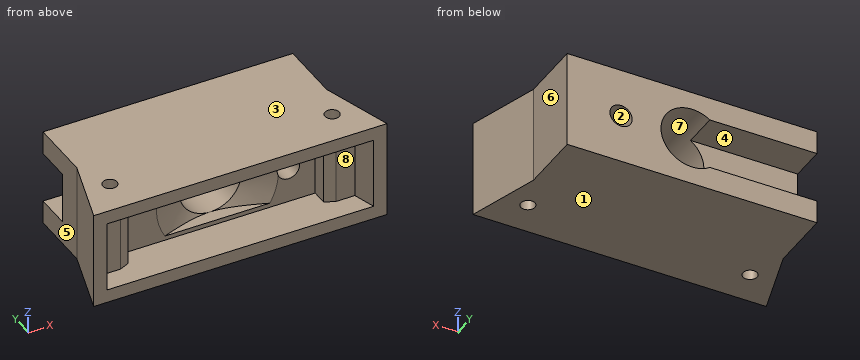
from build123d import *

# Parameters (mm, degrees)
SKETCH1_W                      = 33
SKETCH1_H                      = 11
SKETCH1_W_2                    = 30.000000000000036
SKETCH1_H_2                    = 7.99999999999994
BOSS_EXTRUDE1_DEPTH            = 8
SKETCH3_R                      = 0.8000000000000009
CUT_EXTRUDE3_DEPTH             = 22.383404780343106
CUT_EXTRUDE5_REACH             = 21.144
SKETCH5_R                      = 3.5
CUT_EXTRUDE5_DIRECTION_2_DEPTH = 20.144189719076667
CUT_EXTRUDE4_DEPTH             = 22.383404780343106
CUT_EXTRUDE9_START             = -1.5
CUT_EXTRUDE9_DEPTH             = 8
CUT_EXTRUDE8_DEPTH             = 2.25
BOSS_EXTRUDE8_START            = 3
SKETCH12_W                     = 28.108309096661426
SKETCH12_H                     = 11
SKETCH12_R                     = 3.5
BOSS_EXTRUDE8_DEPTH            = 3
CHAMFER1_SIZE                  = 3.369055161
CHAMFER1_SIZE_2                = 1.5
CHAMFER2_SIZE                  = 0.5
CHAMFER2_SIZE2                 = 1.1230183869521158
CHAMFER3_SIZE                  = 0.5
CHAMFER3_SIZE2                 = 1.1230183869521158
BOSS_EXTRUDE9_REACH            = 20.481
BOSS_EXTRUDE10_START           = 4
BOSS_EXTRUDE10_DEPTH           = 4
CUT_EXTRUDE10_REACH            = 24.967
SKETCH20_R                     = 1.2499999999999991


with BuildPart() as part:
    # Sketch1 → Boss-Extrude1 (new body)
    # profile 1 of 2: a face of its own
    with BuildSketch(Plane(origin=(0, 0, 0), x_dir=(1, 0, 0), z_dir=(0, 1, 0))):
        Rectangle(SKETCH1_W, SKETCH1_H)
        Rectangle(SKETCH1_W_2, SKETCH1_H_2, mode=Mode.SUBTRACT)
    # profile 2 of 2: a face of its own
    with BuildSketch(Plane(origin=(0, 0, 0), x_dir=(1, 0, 0), z_dir=(0, 1, 0))):
        Rectangle(SKETCH1_W_2, SKETCH1_H_2)
    extrude(amount=BOSS_EXTRUDE1_DEPTH)

    # Sketch3 → Cut-Extrude3 (cut, through all)
    with BuildSketch(Plane.XY.offset(5.50000000000003)):
        with Locations((-12.500000000000014, 4)):
            Circle(SKETCH3_R)
        with Locations((12.499999999999988, 4)):
            Circle(SKETCH3_R)
    extrude(amount=-CUT_EXTRUDE3_DEPTH, mode=Mode.SUBTRACT)

    # Sketch5 → Cut-Extrude5 (cut, up to next)
    with BuildSketch(Plane(origin=(0, 8, 0), x_dir=(1, 0, 0), z_dir=(0, 1, 0)), mode=Mode.PRIVATE) as cut_extrude5_sk1:
        with Locations(Location((0, 0, 0), (0, 0, 90))):
            Circle(SKETCH5_R)
    cut_extrude5_tool1 = extrude(cut_extrude5_sk1.sketch, amount=-CUT_EXTRUDE5_REACH, mode=Mode.PRIVATE) & part.part
    add(cut_extrude5_tool1.solids().sort_by_distance((0, 8, 0))[0], mode=Mode.SUBTRACT)

    # Sketch5 → Cut-Extrude5 direction 2 (cut)
    with BuildSketch(Plane(origin=(0, 8, 0), x_dir=(1, 0, 0), z_dir=(0, 1, 0))):
        with Locations(Location((0, 0, 0), (0, 0, 90))):
            Circle(SKETCH5_R)
    extrude(amount=CUT_EXTRUDE5_DIRECTION_2_DEPTH, mode=Mode.SUBTRACT)

    # Sketch4 → Cut-Extrude4 (cut, through all)
    with BuildSketch(Plane.XY.offset(5.50000000000003)):
        Polygon((-16.500000000000014, 0), (-14.054154548330727, 8), (-16.500000000000014, 8), align=None)
        Polygon((16.499999999999986, 0), (14.0541545483307, 8), (16.499999999999986, 8), align=None)
    extrude(amount=-CUT_EXTRUDE4_DEPTH, mode=Mode.SUBTRACT)

    # Sketch14 → Cut-Extrude9 (cut)
    with BuildSketch(Plane.XY.offset(5.50000000000003).offset(CUT_EXTRUDE9_START)):
        Polygon((-15.000000000000014, 0), (14.999999999999988, 0), (14.23567329635332, 2.5000000000000067), (-14.235673296353353, 2.500000000000003), align=None)
    extrude(amount=-CUT_EXTRUDE9_DEPTH, mode=Mode.SUBTRACT)

    # Sketch9 → Cut-Extrude8 (cut)
    with BuildSketch(Plane.XZ.offset(-2.500000000000005)):
        Polygon((-11.000000000000002, 4.000000000000002), (11.000000000000002, 4.000000000000001), (11.000000000000004, -3.999999999999999), (-11, -4.000000000000002), align=None)
    extrude(amount=-CUT_EXTRUDE8_DEPTH, mode=Mode.SUBTRACT)

    # Sketch12 → Boss-Extrude8 (add)
    with BuildSketch(Plane(origin=(0, 8, 0), x_dir=(1, 0, 0), z_dir=(0, 1, 0)).offset(BOSS_EXTRUDE8_START)):
        Rectangle(SKETCH12_W, SKETCH12_H)
        with Locations(Location((0, 0, 0), (0, 0, 90))):
            Circle(SKETCH12_R, mode=Mode.SUBTRACT)
    extrude(amount=-BOSS_EXTRUDE8_DEPTH)

    # Chamfer1
    # the kernel refuses this chamfer: 3.369055161, 1.5 mm, written as the material it takes off along each edge
    with BuildSketch(Plane(origin=(0, 4.750000000000005, 0), x_dir=(6e-17, 0, -1), z_dir=(1, 0, 6e-17))) as chamfer1_piece_1_section:
        Polygon((3.5 + CHAMFER1_SIZE, 0), (3.5, CHAMFER1_SIZE_2), (3.5, 0), align=None)
    chamfer1_piece_1 = revolve(axis=Axis((0, 4.750000000000005, 0), (0, 1, 0)), mode=Mode.PRIVATE)
    chamfer1_piece_1 = split(chamfer1_piece_1, bisect_by=Plane(origin=(-5.449382074907194, 4.96599151817854, 4.00000000000003), z_dir=(0, 0, -1)), keep=Keep.TOP, mode=Mode.PRIVATE)
    chamfer1_piece_1 = split(chamfer1_piece_1, bisect_by=Plane(origin=(-5.449382074907194, 4.96599151817854, -3.99999999999997), z_dir=(0, 0, 1)), keep=Keep.TOP, mode=Mode.PRIVATE)
    add(chamfer1_piece_1, mode=Mode.SUBTRACT)

    # Chamfer2
    chamfer2_edges = [part.edges().sort_by_distance(p)[0] for p in [
        (-11, 2.5000000000000036, 0),
    ]]
    chamfer2_side = [part.faces().sort_by_distance(p)[0] for p in [
        (-11.000000000000002, 3.625000000000003, 0),
    ]]
    chamfer(chamfer2_edges, length=CHAMFER2_SIZE, length2=CHAMFER2_SIZE2, reference=chamfer2_side[0])

    # Chamfer3
    chamfer3_edges = [part.edges().sort_by_distance(p)[0] for p in [
        (11.000000000000004, 2.500000000000006, 8.9e-16),
    ]]
    chamfer3_side = [part.faces().sort_by_distance(p)[0] for p in [
        (11.000000000000002, 3.625000000000006, 7.9e-16),
    ]]
    chamfer(chamfer3_edges, length=CHAMFER3_SIZE, length2=CHAMFER3_SIZE2, reference=chamfer3_side[0])

    # Sketch17 → Boss-Extrude9 (add, up to next)
    with BuildSketch(Plane.XZ.offset(-4.750000000000004), mode=Mode.PRIVATE) as boss_extrude9_sk1:
        Polygon((5.910492264007006, -3.500000000000001), (8.9e-16, -3.5), (-5.910492264007006, -3.500000000000001), (-5.910492264007006, -3.999999999999969), (5.910492264007006, -3.999999999999969), align=None)
    boss_extrude9_tool1 = extrude(boss_extrude9_sk1.sketch, amount=-BOSS_EXTRUDE9_REACH, mode=Mode.PRIVATE) - part.part
    add(boss_extrude9_tool1.solids().sort_by_distance((0, 4.75, -3.75))[0])

    # Sketch18 → Boss-Extrude10 (add)
    with BuildSketch(Plane(origin=(0, 11, 0), x_dir=(1, 0, 0), z_dir=(0, 1, 0)).offset(BOSS_EXTRUDE10_START)):
        with BuildLine():
            Line((-1.9960899278338715, -2.875000000000029), (-14.054154548330727, -2.875000000000029))
            Line((-14.054154548330727, -2.875000000000029), (-14.054154548330727, -5.50000000000003))
            Line((-14.054154548330729, -5.50000000000003), (14.0541545483307, -5.50000000000003))
            Line((14.0541545483307, -5.50000000000003), (14.0541545483307, -2.875000000000029))
            Line((14.054154548330702, -2.875000000000029), (1.9960899278337951, -2.875000000000029))
            ThreePointArc((1.996089927833807, -2.8750000000000746), (-3.947e-14, -3.5), (-1.9960899278338722, -2.8750000000000293))
        make_face()
        with BuildLine():
            Line((14.0541545483307, 5.499999999999971), (-14.054154548330729, 5.499999999999971))
            Line((-14.054154548330727, 5.499999999999971), (-14.054154548330727, 2.8749999999999707))
            Line((-14.054154548330727, 2.8749999999999707), (-1.9960899278339532, 2.8749999999999707))
            ThreePointArc((-1.996089927833954, 2.8749999999999725), (-4.946e-14, 3.5), (1.9960899278338722, 2.875000000000029))
            Line((1.9960899278338768, 2.8749999999999702), (14.054154548330702, 2.8749999999999702))
            Line((14.0541545483307, 2.8749999999999702), (14.0541545483307, 5.499999999999971))
        make_face()
        with BuildLine():
            Line((14.0541545483307, -2.875000000000029), (14.0541545483307, 2.87499999999997))
            Line((14.054154548330702, 2.8749999999999702), (1.9960899278338768, 2.8749999999999702))
            ThreePointArc((1.9960899278338722, 2.875000000000029), (3.1013154263488385, 1.6222954805739687), (3.5000000000000004, 0))
            ThreePointArc((3.5000000000000004, 0), (3.10131542634882, -1.622295480574004), (1.996089927833807, -2.8750000000000746))
            Line((1.9960899278337951, -2.875000000000029), (14.054154548330702, -2.875000000000029))
        make_face()
    extrude(amount=-BOSS_EXTRUDE10_DEPTH)

    # Sketch20 → Cut-Extrude10 (cut, up to next)
    with BuildSketch(Plane(origin=(0, 15, 0), x_dir=(1, 0, 0), z_dir=(0, 1, 0)), mode=Mode.PRIVATE) as cut_extrude10_sk1:
        with Locations(Location((8, 0, 0), (0, 0, 270))):
            Circle(SKETCH20_R)
    cut_extrude10_tool1 = extrude(cut_extrude10_sk1.sketch, amount=-CUT_EXTRUDE10_REACH, mode=Mode.PRIVATE) & part.part
    add(cut_extrude10_tool1.solids().sort_by_distance((8, 15, 0))[0], mode=Mode.SUBTRACT)


solid = part.part
Read the model definition and answer for the solid it produces. Units are mm, in the model's axes. Face numbers are marked on the shaded views. A direction names the side the tool comes from. Round coordinates to 2 decimals unless told otherwise and drop trailing zeros. Write each loop counter-clockwise with the first axis right and the second up, starting at its lowest first coordinate (ties: lowest second). Pieces come first, ordered by that corner, then holes.
Q1. Flat-ended cylindrical pins translate along their axes: P1, Ø4, axis at y = 13, z = 2, coming from the +X side; P2, Ø1.1, axis at x = 13.5, z = -1.5, coming from the -Y side; P3, Ø1.8, axis at x = 12.5, y = 4, coming from the -Z side; P4, Ø1.9, axis at y = 4, z = -0.5, coming from the -X side. Find the tip coordinate at first contact, or state that the pin passes through.
Values:
P1: stops at x = 14.05
P2: stops at y = 2.5
P3: stops at z = -5.5
P4: stops at x = -15.57
Q2. Find section B-B on y = 12.75. Determine the outline of the cut face in (x, z) (3 decimals).
Values:
outline: (-14.054, -5.5) - (14.054, -5.5) - (14.054, 5.5) - (-14.054, 5.5) - (-14.054, 2.875) - (-1.996, 2.875) arc R3.5 cw (long way) to (-1.996, -2.875) - (-14.054, -2.875) - close; hole circle Ø2.5 at (8, 0)
Q3. The mould has two halves that part along Z. Classify the marked faces 1, 2 and 3: released by +Z, released by -Z, zero draft, split by the parting line, or undercut.
Values:
face 1: released by -Z
face 2: undercut
face 3: released by +Z
Q4. Find section A-A on x = 12.5. Determine the outline of the cut face in (y, z), and give its area (3 significant figures).
Values:
outline: (0, -5.5) - (3.2, -5.5) - (3.2, 5.5) - (0, 5.5) - (0, 4) - (2.5, 4) - (2.5, -4) - (0, -4) - close; (4.8, -5.5) - (15, -5.5) - (15, 5.5) - (4.8, 5.5) - close
area: 127 mm2
Q5. Find section D-D on x = -8. Determine the outline of the cut face in (y, z) (3 decimals), and give its area (3 significant figures).
Values:
outline: (0, -5.5) - (15, -5.5) - (15, -2.875) - (11, -2.875) - (11, 2.875) - (15, 2.875) - (15, 5.5) - (0, 5.5) - (0, 4) - (4.75, 4) - (4.75, -4) - (0, -4) - close
area: 104 mm2
Q6. Find section C-C on z = 4.5. Determine the outline of the cut face in (x, y), and give its area (3 significant figures).
Values:
outline: (-16.5, 0) - (16.5, 0) - (14.05, 8) - (14.05, 15) - (-14.05, 15) - (-14.05, 8) - close; hole circle Ø1.6 at (-12.5, 4); hole circle Ø1.6 at (12.5, 4)
area: 437 mm2
Q7. Straight lines are drawn through the part: line 1 (X direction, y = 10, z = 0); line 2 (Z direction, x = -0.5, y = 4.25); line 3 (Z direction, x = 8, y = 7). For each, find the intervals that lie inside material, in ascending order.
Values:
line 1: x = -14.05 to -3.5, 3.5 to 6.75, 9.25 to 14.05
line 2: z = -5.5 to -4, 4 to 5.5
line 3: z = -5.5 to -1.25, 1.25 to 5.5
Q8. A tool of negligible diameter and unlimited length cuts with its end or side. For the marked faces 4, 5, 6, 7 and 8, from which of +Z, -Z, +X, -X, +Y, -Y can it reach the whole face along a straight path? Write none if from no direction.
Values:
face 4: -X, +Y
face 5: +Z, -Z, -X, +Y
face 6: +Z, -Z, +X, +Y
face 7: +Y, -Y
face 8: -Y
